CAD build for the part. Positions are in the model's coordinates, mm. A direction names the side the tool comes from. Give positions to 0.01 mm unless a question says otherwise; leave off trailing zeros. Order: outer loops, then holes, each group sorted by start corner. A loop starts at its lowest first (then second) coordinate and runs counter-clockwise, first axis right, second up. Notation, with made-up numbers: (-31.5, 66) -> (10.5, 66) arc R18 cw to (10.5, 95) -> close; hole circle Ø2 at (-33.75, 60.25). An arc over 180 degrees is marked (long way). Answer as CSV lines item,"result".
```python
from build123d import *

# Parameters (mm, degrees)
OUTER_RACE_KEEPER_FLANGE_PROFILE_R             = 17
OUTER_RACE_KEEPER_FLANGE_DEPTH                 = 2
HOUSING_CONTACT_RIM_PRESERVES_BEARING_FL_START = -0.2
HOUSING_CONTACT_RIM_PRESERVES_BEARIN_2_R       = 17
HOUSING_CONTACT_RIM_PRESERVES_BEARIN_2_R_2     = 11.2
HOUSING_CONTACT_RIM_PRESERVES_BEARING_FL_DEPTH = 0.2
PIN_END_COVER_PROFILE_R                        = 9
PIN_END_COVER_DEPTH                            = 12
DOWEL_END_FLOAT_POCKET_PROFILE_R               = 7
DOWEL_END_FLOAT_POCKET_DEPTH9_DEPTH            = 9
KEEPER_M2_FASTENERS_START                      = -50
KEEPER_M2_FASTENERS_PROFILE_R                  = 1.1
KEEPER_M2_FASTENERS_DEPTH                      = 77.870057685


with BuildPart() as part:
    # Outer_race_keeper_flange_profile → Outer_race_keeper_flange (new body)
    with BuildSketch(Plane.XY):
        Circle(OUTER_RACE_KEEPER_FLANGE_PROFILE_R)
    extrude(amount=OUTER_RACE_KEEPER_FLANGE_DEPTH)

    # Housing_contact_rim_preserves_bearin 2 → Housing_contact_rim_preserves_bearing_fl (add)
    with BuildSketch(Plane.XY.offset(HOUSING_CONTACT_RIM_PRESERVES_BEARING_FL_START)):
        Circle(HOUSING_CONTACT_RIM_PRESERVES_BEARIN_2_R)
        Circle(HOUSING_CONTACT_RIM_PRESERVES_BEARIN_2_R_2, mode=Mode.SUBTRACT)
    extrude(amount=HOUSING_CONTACT_RIM_PRESERVES_BEARING_FL_DEPTH)

    # Pin_end_cover_profile → Pin_end_cover (add)
    with BuildSketch(Plane.XY):
        Circle(PIN_END_COVER_PROFILE_R)
    extrude(amount=PIN_END_COVER_DEPTH)

    # Dowel_end_float_pocket_profile → Dowel_end_float_pocket_depth9 (cut)
    with BuildSketch(Plane.XY):
        Circle(DOWEL_END_FLOAT_POCKET_PROFILE_R)
    extrude(amount=DOWEL_END_FLOAT_POCKET_DEPTH9_DEPTH, mode=Mode.SUBTRACT)

    # Keeper_M2_fasteners_profile → Keeper_M2_fasteners (cut, through all)
    with BuildSketch(Plane.XY.offset(KEEPER_M2_FASTENERS_START)):
        with Locations((14, 0)):
            Circle(KEEPER_M2_FASTENERS_PROFILE_R)
        with Locations((0, -14)):
            Circle(KEEPER_M2_FASTENERS_PROFILE_R)
        with Locations((0, 14)):
            Circle(KEEPER_M2_FASTENERS_PROFILE_R)
    extrude(amount=KEEPER_M2_FASTENERS_DEPTH, mode=Mode.SUBTRACT)


solid = part.part
```
1) Wall check: line 1 along Y through (x, z) = (0, 4.5); line 2 along Z through (x, y) = (10.5, 0); line 3 along Z through (x, y) = (-14, 3). Give the ranges that are in metal, low to high. Write a range as [from, to].
Data:
line 1,"y = [-9, -7], [7, 9]"
line 2,"z = [0, 2]"
line 3,"z = [-0.2, 2]"
2) Pin check, flat tips, straight feed: P1, Ø4, axis at y = 12.5, z = 2, coming from the +X side; P2, Ø6, axis at x = -4.5, y = 3.5, coming from the -Z side; P3, Ø13.5, axis at x = 0, y = 0, coming from the -Z side; P4, Ø1.3, axis at x = 0, y = 14, coming from the +Z side. Stop position of each tip, or through.
Data:
P1,"stops at x = 13.37"
P2,"stops at z = 0"
P3,"stops at z = 9"
P4,"passes through"
3) Band-saw the part on A-A, the plane y = 0. Write the cut outline in (x, z), then the cut area to 3 significant figures.
Data:
outline,"(-17, -0.2) -> (-11.2, -0.2) -> (-11.2, 0) -> (-7, 0) -> (-7, 9) -> (7, 9) -> (7, 0) -> (11.2, 0) -> (11.2, -0.2) -> (12.9, -0.2) -> (12.9, 2) -> (9, 2) -> (9, 12) -> (-9, 12) -> (-9, 2) -> (-17, 2) -> close; (15.1, -0.2) -> (17, -0.2) -> (17, 2) -> (15.1, 2) -> close"
area,"119 mm2"
4) Band-saw the part on C-C, the plane x = 0. Write the cut outline in (y, z), then the cut area to 3 significant figures.
Data:
outline,"(-17, -0.2) -> (-15.1, -0.2) -> (-15.1, 2) -> (-17, 2) -> close; (-12.9, -0.2) -> (-11.2, -0.2) -> (-11.2, 0) -> (-7, 0) -> (-7, 9) -> (7, 9) -> (7, 0) -> (11.2, 0) -> (11.2, -0.2) -> (12.9, -0.2) -> (12.9, 2) -> (9, 2) -> (9, 12) -> (-9, 12) -> (-9, 2) -> (-12.9, 2) -> close; (15.1, -0.2) -> (17, -0.2) -> (17, 2) -> (15.1, 2) -> close"
area,"115 mm2"
5) Which spindle directions (+Z, -Z, +X, -X, +Y, -Y) get a long thin tool onto all of the face, cutting with end or side? Do faces 4 (the cylindrical face through (-0.238, 12.926, 0.885)), 5 (the flat face through (7, -7, 2)), 6 (the flat face through (0, 0, 9)). Say none if no direction does.
Data:
face 4,"+Z, -Z"
face 5,"+Z"
face 6,"-Z"
6) Band-saw the part on B-B, the plane z = 1.5. Write the cut outline in (x, y).
Data:
outline,"circle Ø34 at (0, 0); hole circle Ø14 at (0, 0); hole circle Ø2.2 at (0, -14); hole circle Ø2.2 at (0, 14); hole circle Ø2.2 at (14, 0)"
7) Pull direction X, two halves, no side cores. Call faces 1 (the cylindrical face through (-1.172, 8.923, 6.93)), 2 (the flat face through (0, 0, 12)), 3 (the cylindrical face through (12.9, 0, 0.9)): pulls with the +X half, pulls with the -X half, needs draft (parallel to the pull), parting line crosses it, or undercut.
Data:
face 1,"parting line crosses it"
face 2,"needs draft"
face 3,"undercut"
8) Band-saw the part on D-D, the plane x = 14. Write the cut outline in (y, z), then the cut area to 3 significant figures.
Data:
outline,"(-9.64, -0.2) -> (-1.1, -0.2) -> (-1.1, 2) -> (-9.64, 2) -> close; (1.1, -0.2) -> (9.64, -0.2) -> (9.64, 2) -> (1.1, 2) -> close"
area,"37.6 mm2"
